Geometry: final body of the model. Coordinates: model frame, mm. Face numbers are marked on the shaded views. A direction names the side the tool comes from. Round coordinates to 2 decimals unless told otherwise and drop trailing zeros. Order: outer loops, then holes, each group sorted by start corner. A loop starts at its lowest first (then second) coordinate and runs counter-clockwise, first axis right, second up. Notation, with made-up numbers: (54.25, -18) - (110.25, -18) arc R23 ccw to (110.25, 8) - close; hole circle Ø10 at (67, -4). An arc over 180 degrees is marked (long way). Put each result on its own line as item: value. Start each with the question number.
(1) Section C-C (z = -10.5). Output: boundary loops of the cut face in (x, y), and give its area (3 significant figures).
(2) Pin query (flat end, axial travel): P1, Ø1, axis at x = 30, y = 8, coming from the +Z side; P2, Ø8, axis at x = 11, y = -10.5, coming from the -Z side; P3, Ø5, axis at x = 42, z = 14.5, coming from the -Y side. Return the tip coordinate at first contact, or that it passes through.
(3) Section D-D (y = -38). Output: boundary loops of the cut face in (x, z), and give its area (3 significant figures).
(4) Material intervals for L1, parallel to X at y = 11.5, z = -61.5; L2, parallel to Y at x = 41, z = 19.5; L3, parallel to Z at x = 43, y = -18, sorted ascending. Write a range as [from, to].
(5) Pull-direction query (Y, two-part tool) for the marked faces 5, 6, 7 and 8; classes: released by +Y, released by -Y, zero draft, split by the parting line, or undercut.
(6) Section B-B (x = 40). Count the separate pieces of the cut face and the enclosed holes in it, and give its area (3 significant figures).
(7) Section A-A (y = 6). Output: boundary loops of the cut face in (x, z).
(8) Access query for the marked faces 1, 2, 3 and 4. Directions: +Z, -Z, +X, -X, +Y, -Y. A direction counts if a zero-diameter tool reaches every point of the face in a straight line with its end or side. Return the directions, or none.
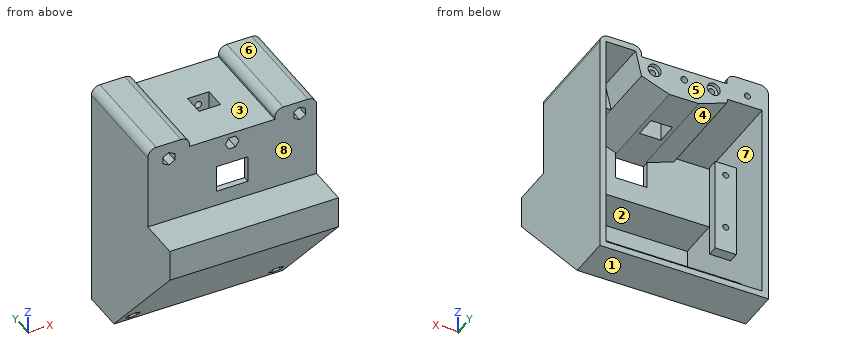
from build123d import *

# Parameters (mm, degrees)
BOSS_EXTRUDE1_DEPTH = 80
SHELL1_T            = -3
SKETCH3_W           = 46
SKETCH3_H           = 47
BOSS_EXTRUDE2_DEPTH = 17
SKETCH4_W           = 10.2
SKETCH4_H           = 10.2
CUT_EXTRUDE1_DEPTH  = 20
SKETCH6_W           = 15
SKETCH6_H           = 12.8
CUT_EXTRUDE2_DEPTH  = 3
SKETCH7_W           = 40.4
SKETCH7_H           = 50
CUT_EXTRUDE3_DEPTH  = 5
FILLET1_R           = 4
CUT_EXTRUDE7_DEPTH  = 47
SKETCH13_R          = 1.5
CUT_EXTRUDE8_DEPTH  = 25
SKETCH14_R          = 3.1
CUT_EXTRUDE9_DEPTH  = 2
SKETCH17_W          = 45
SKETCH17_H          = 5
BOSS_EXTRUDE5_DEPTH = 74
CUT_EXTRUDE10_REACH = 126.093
SKETCH18_W          = 54
SKETCH18_H          = 45
CUT_EXTRUDE11_REACH = 126.093
SKETCH19_R          = 1.45
BOSS_EXTRUDE6_DEPTH = 47
SKETCH22_R          = 1.45
CUT_EXTRUDE12_DEPTH = 135.415364765
BOSS_EXTRUDE7_DEPTH = 74
SKETCH27_R          = 1.65
CUT_EXTRUDE14_DEPTH = 10
CUT_EXTRUDE15_START = -3
CUT_EXTRUDE15_DEPTH = 32
CUT_EXTRUDE16_DEPTH = 30
BOSS_EXTRUDE8_DEPTH = 20
SKETCH31_R          = 1.5
CUT_EXTRUDE17_DEPTH = 123.649786567
CUT_EXTRUDE18_DEPTH = 15
CUT_EXTRUDE19_REACH = 126.093
SKETCH33_W          = 10
SKETCH33_H          = 5
SKETCH34_R          = 1.6
CUT_EXTRUDE20_DEPTH = 135.415364765
CUT_EXTRUDE22_DEPTH = 14


with BuildPart() as part:
    # Sketch2 → Boss-Extrude1 (new body)
    with BuildSketch(Plane(origin=(0, 0, 0), x_dir=(0, 0, -1), z_dir=(1, 0, 0))):
        Polygon((-27.320490368, 20.998248687), (-27.320490368, -29.001751313), (12.679509632, -29.001751313), (12.679509632, -48.511383538), (27.679509632, -48.511383538), (82.679509632, 0.998248687), (82.679509632, 20.998248687), align=None)
    extrude(amount=BOSS_EXTRUDE1_DEPTH)

    # Shell1
    shell1_openings = [part.faces().sort_by_distance(p)[0] for p in [
        (40, 20.998248687, -27.679509632),
    ]]
    offset(amount=SHELL1_T, openings=shell1_openings, kind=Kind.INTERSECTION)

    # Sketch3 → Boss-Extrude2 (add)
    with BuildSketch(Plane(origin=(0, 0, 24.320490368), x_dir=(-1, 0, 0), z_dir=(0, 0, -1))):
        with Locations((-40, -2.501751313)):
            Rectangle(SKETCH3_W, SKETCH3_H)
    extrude(amount=BOSS_EXTRUDE2_DEPTH)

    # Sketch4 → Cut-Extrude1 (cut)
    with BuildSketch(Plane.XY.offset(27.320490368)):
        with Locations((40, -4.001751313)):
            Rectangle(SKETCH4_W, SKETCH4_H)
    extrude(amount=-CUT_EXTRUDE1_DEPTH, mode=Mode.SUBTRACT)

    # Sketch6 → Cut-Extrude2 (cut)
    with BuildSketch(Plane.XZ.offset(29.001751313)):
        with Locations((40, 0.920490368)):
            Rectangle(SKETCH6_W, SKETCH6_H)
    extrude(amount=-CUT_EXTRUDE2_DEPTH, mode=Mode.SUBTRACT)

    # Sketch7 → Cut-Extrude3 (cut)
    with BuildSketch(Plane.XY.offset(27.320490368)):
        with Locations((40, -4.001751313)):
            Rectangle(SKETCH7_W, SKETCH7_H)
    extrude(amount=-CUT_EXTRUDE3_DEPTH, mode=Mode.SUBTRACT)

    # Fillet1
    fillet1_edges = [part.edges().sort_by_distance(p)[0] for p in [
        (80, -4.001751313, 27.320490368),
        (19.8, -4.001751313, 27.320490368),
        (0, -4.001751313, 27.320490368),
        (60.2, -4.001751313, 27.320490368),
    ]]
    fillet(fillet1_edges, radius=FILLET1_R)

    # Sketch12 → Cut-Extrude7 (cut)
    with BuildSketch(Plane(origin=(0, 20.998248687, 0), x_dir=(1, 0, 0), z_dir=(0, 1, 0))):
        Polygon((33, -7.320490368), (19.8, -12.320490368), (17, -24.320490368), (17, -7.320490368), align=None)
        Polygon((47, -7.320490368), (63, -7.320490368), (63, -24.320490368), (60.2, -12.320490368), align=None)
    extrude(amount=-CUT_EXTRUDE7_DEPTH, mode=Mode.SUBTRACT)

    # Sketch13 → Cut-Extrude8 (cut)
    with BuildSketch(Plane(origin=(0, 20.998248687, 0), x_dir=(1, 0, 0), z_dir=(0, 1, 0))):
        with Locations(Location((26, -17.320490368, 0), (0, 0, 270))):
            Circle(SKETCH13_R)
        with Locations(Location((54, -17.320490368, 0), (0, 0, 270))):
            Circle(SKETCH13_R)
    extrude(amount=-CUT_EXTRUDE8_DEPTH, mode=Mode.SUBTRACT)

    # Sketch14 → Cut-Extrude9 (cut)
    with BuildSketch(Plane(origin=(0, 20.998248687, 0), x_dir=(1, 0, 0), z_dir=(0, 1, 0))):
        with Locations(Location((26, -17.320490368, 0), (0, 0, 270))):
            Circle(SKETCH14_R)
        with Locations(Location((54, -17.320490368, 0), (0, 0, 270))):
            Circle(SKETCH14_R)
    extrude(amount=-CUT_EXTRUDE9_DEPTH, mode=Mode.SUBTRACT)

    # Sketch17 → Boss-Extrude5 (add)
    with BuildSketch(Plane.ZY.offset(-77)):
        with Locations((-23.179509632, -4.501751313)):
            Rectangle(SKETCH17_W, SKETCH17_H)
    extrude(amount=BOSS_EXTRUDE5_DEPTH)

    # Sketch18 → Cut-Extrude10 (cut, up to next)
    with BuildSketch(Plane(origin=(0, -2.001751313, 0), x_dir=(1, 0, 0), z_dir=(0, 1, 0)), mode=Mode.PRIVATE) as cut_extrude10_sk1:
        with Locations((40, 23.179509632)):
            Rectangle(SKETCH18_W, SKETCH18_H)
    cut_extrude10_tool1 = extrude(cut_extrude10_sk1.sketch, amount=-CUT_EXTRUDE10_REACH, mode=Mode.PRIVATE) & part.part
    add(cut_extrude10_tool1.solids().sort_by_distance((40, -2.001751, -23.17951))[0], mode=Mode.SUBTRACT)

    # Sketch19 → Cut-Extrude11 (cut, up to next)
    with BuildSketch(Plane(origin=(0, -2.001751313, 0), x_dir=(1, 0, 0), z_dir=(0, 1, 0)), mode=Mode.PRIVATE) as cut_extrude11_sk1:
        with Locations(Location((72, 37.179509632, 0), (0, 0, 270))):
            Circle(SKETCH19_R)
    cut_extrude11_tool1 = extrude(cut_extrude11_sk1.sketch, amount=-CUT_EXTRUDE11_REACH, mode=Mode.PRIVATE) & part.part
    # Sketch19 → Cut-Extrude11 (cut, up to next)
    with BuildSketch(Plane(origin=(0, -2.001751313, 0), x_dir=(1, 0, 0), z_dir=(0, 1, 0)), mode=Mode.PRIVATE) as cut_extrude11_sk2:
        with Locations(Location((72, 6.179509632, 0), (0, 0, 270))):
            Circle(SKETCH19_R)
    cut_extrude11_tool2 = extrude(cut_extrude11_sk2.sketch, amount=-CUT_EXTRUDE11_REACH, mode=Mode.PRIVATE) & part.part
    # Sketch19 → Cut-Extrude11 (cut, up to next)
    with BuildSketch(Plane(origin=(0, -2.001751313, 0), x_dir=(1, 0, 0), z_dir=(0, 1, 0)), mode=Mode.PRIVATE) as cut_extrude11_sk3:
        with Locations(Location((8, 33.179509632, 0), (0, 0, 270))):
            Circle(SKETCH19_R)
    cut_extrude11_tool3 = extrude(cut_extrude11_sk3.sketch, amount=-CUT_EXTRUDE11_REACH, mode=Mode.PRIVATE) & part.part
    # Sketch19 → Cut-Extrude11 (cut, up to next)
    with BuildSketch(Plane(origin=(0, -2.001751313, 0), x_dir=(1, 0, 0), z_dir=(0, 1, 0)), mode=Mode.PRIVATE) as cut_extrude11_sk4:
        with Locations(Location((8, 6.179509632, 0), (0, 0, 270))):
            Circle(SKETCH19_R)
    cut_extrude11_tool4 = extrude(cut_extrude11_sk4.sketch, amount=-CUT_EXTRUDE11_REACH, mode=Mode.PRIVATE) & part.part
    add(cut_extrude11_tool1.solids().sort_by_distance((72, -2.001751, -37.17951))[0], mode=Mode.SUBTRACT)
    add(cut_extrude11_tool2.solids().sort_by_distance((72, -2.001751, -6.17951))[0], mode=Mode.SUBTRACT)
    add(cut_extrude11_tool3.solids().sort_by_distance((8, -2.001751, -33.17951))[0], mode=Mode.SUBTRACT)
    add(cut_extrude11_tool4.solids().sort_by_distance((8, -2.001751, -6.17951))[0], mode=Mode.SUBTRACT)

    # Sketch21 → Boss-Extrude6 (add)
    with BuildSketch(Plane(origin=(0, -26.001751313, 0), x_dir=(1, 0, 0), z_dir=(0, 1, 0))):
        Polygon((3, -24.320490368), (3, -14.320490368), (19.333333333, -14.320490368), (17, -24.320490368), align=None)
    extrude(amount=BOSS_EXTRUDE6_DEPTH)

    # Sketch22 → Cut-Extrude12 (cut, through all)
    with BuildSketch(Plane(origin=(0, 20.998248687, 0), x_dir=(1, 0, 0), z_dir=(0, 1, 0))):
        with Locations(Location((10, -19.320490368, 0), (0, 0, 270))):
            Circle(SKETCH22_R)
    extrude(amount=-CUT_EXTRUDE12_DEPTH, mode=Mode.SUBTRACT)

    # Sketch26 → Boss-Extrude7 (add)
    with BuildSketch(Plane(origin=(3, 0, 0), x_dir=(0, 0, -1), z_dir=(1, 0, 0))):
        Polygon((79.679509632, 2.334161996), (63.679509632, 2.334161996), (63.679509632, -12.068640106), align=None)
    extrude(amount=BOSS_EXTRUDE7_DEPTH)

    # Sketch27 → Cut-Extrude14 (cut)
    with BuildSketch(Plane(origin=(0, 2.334161996, 0), x_dir=(1, 0, 0), z_dir=(0, 1, 0))):
        with Locations(Location((6, 76.679509632, 0), (0, 0, 270))):
            Circle(SKETCH27_R)
        with Locations(Location((74, 76.679509632, 0), (0, 0, 270))):
            Circle(SKETCH27_R)
    extrude(amount=-CUT_EXTRUDE14_DEPTH, mode=Mode.SUBTRACT)

    # Sketch28 → Cut-Extrude15 (cut)
    with BuildSketch(Plane(origin=(0, 2.334161996, 0), x_dir=(1, 0, 0), z_dir=(0, 1, 0)).offset(CUT_EXTRUDE15_START)):
        Polygon((74, 79.929509632), (71.185417438, 78.304509632), (71.185417438, 75.054509632), (74, 73.429509632), (76.814582562, 75.054509632), (76.814582562, 78.304509632), align=None)
        Polygon((6, 73.429509632), (8.814582562, 75.054509632), (8.814582562, 78.304509632), (6, 79.929509632), (3.185417438, 78.304509632), (3.185417438, 75.054509632), align=None)
    extrude(amount=-CUT_EXTRUDE15_DEPTH, mode=Mode.SUBTRACT)

    # Sketch29 → Cut-Extrude16 (cut)
    with BuildSketch(Plane.XZ.offset(29.001751313)):
        Polygon((7.185417438, 17.695490368), (10, 16.070490368), (12.814582562, 17.695490368), (12.814582562, 20.945490368), (10, 22.570490368), (7.185417438, 20.945490368), align=None)
    extrude(amount=-CUT_EXTRUDE16_DEPTH, mode=Mode.SUBTRACT)

    # Sketch30 → Boss-Extrude8 (add)
    with BuildSketch(Plane(origin=(0, -26.001751313, 0), x_dir=(1, 0, 0), z_dir=(0, 1, 0))):
        Polygon((77, -24.320490368), (63, -24.320490368), (60.2, -12.320490368), (77, -12.320490368), align=None)
    extrude(amount=BOSS_EXTRUDE8_DEPTH)

    # Sketch31 → Cut-Extrude17 (cut, through all)
    with BuildSketch(Plane(origin=(0, -6.001751313, 0), x_dir=(1, 0, 0), z_dir=(0, 1, 0))):
        with Locations(Location((72, -21.320490368, 0), (0, 0, 270))):
            Circle(SKETCH31_R)
    extrude(amount=-CUT_EXTRUDE17_DEPTH, mode=Mode.SUBTRACT)

    # Sketch32 → Cut-Extrude18 (cut)
    with BuildSketch(Plane.XZ.offset(29.001751313)):
        Polygon((72, 24.570490368), (69.185417438, 22.945490368), (69.185417438, 19.695490368), (72, 18.070490368), (74.814582562, 19.695490368), (74.814582562, 22.945490368), align=None)
    extrude(amount=-CUT_EXTRUDE18_DEPTH, mode=Mode.SUBTRACT)

    # Sketch33 → Cut-Extrude19 (cut, up to next)
    with BuildSketch(Plane(origin=(0, -2.001751313, 0), x_dir=(1, 0, 0), z_dir=(0, 1, 0)), mode=Mode.PRIVATE) as cut_extrude19_sk1:
        with Locations((72, 43.179509632)):
            Rectangle(SKETCH33_W, SKETCH33_H)
    cut_extrude19_tool1 = extrude(cut_extrude19_sk1.sketch, amount=-CUT_EXTRUDE19_REACH, mode=Mode.PRIVATE) & part.part
    add(cut_extrude19_tool1.solids().sort_by_distance((72, -2.001751, -43.17951))[0], mode=Mode.SUBTRACT)

    # Sketch34 → Cut-Extrude20 (cut, through all)
    with BuildSketch(Plane(origin=(0, 20.998248687, 0), x_dir=(1, 0, 0), z_dir=(0, 1, 0))):
        with Locations(Location((40, -17.320490368, 0), (0, 0, 270))):
            Circle(SKETCH34_R)
    extrude(amount=-CUT_EXTRUDE20_DEPTH, mode=Mode.SUBTRACT)

    # Sketch36 → Cut-Extrude22 (cut)
    with BuildSketch(Plane.XZ.offset(29.001751313)):
        Polygon((38.375, 20.13507293), (36.75, 17.320490368), (38.375, 14.505907805), (41.625, 14.505907805), (43.25, 17.320490368), (41.625, 20.13507293), align=None)
    extrude(amount=-CUT_EXTRUDE22_DEPTH, mode=Mode.SUBTRACT)


solid = part.part
Checks:
1. outline: (0, -29) - (80, -29) - (80, 21) - (77, 21) - (77, -2) - (67, -2) - (67, -7) - (77, -7) - (77, -26) - (3, -26) - (3, -7) - (13, -7) - (13, -2) - (3, -2) - (3, 21) - (0, 21) - close
1. area: 622 mm²
2. P1: stops at z = 22.32
2. P2: stops at z = -74.35
2. P3: stops at y = -29
3. outline: (0, -39.36) - (80, -39.36) - (80, -12.68) - (0, -12.68) - close; hole (3, -34.87) - (77, -34.87) - (77, -15.68) - (3, -15.68) - close
3. area: 714 mm²
4. L1: x = [0, 3], [77, 80]
4. L2: y = [-15, -9.1], [1.1, 21]
4. L3: z = [-61.57, -57.09], [7.32, 16.89], [17.75, 22.32]
5. face 5: released by +Y
5. face 6: zero draft
5. face 7: undercut
5. face 8: released by -Y
6. separate pieces: 5
6. enclosed holes: 0
6. area: 951 mm²
7. outline: (0, -82.68) - (80, -82.68) - (80, 23.32) arc R4 ccw to (76, 27.32) - (64.2, 27.32) arc R4 ccw to (60.2, 23.32) - (60.2, 22.32) - (19.8, 22.32) - (19.8, 23.32) arc R4 ccw to (15.8, 27.32) - (4, 27.32) arc R4 ccw to (0, 23.32) - close; hole (3, -79.68) - (77, -79.68) - (77, 24.32) - (63, 24.32) - (60.2, 12.32) - (47, 7.32) - (33, 7.32) - (19.8, 12.32) - (19.33, 14.32) - (3, 14.32) - close; hole circle Ø2.9 at (10, 19.32); hole circle Ø3 at (26, 17.32); hole circle Ø3.2 at (40, 17.32); hole circle Ø3 at (54, 17.32)
8. face 1: -Z, +X, -X, +Y, -Y
8. face 2: none
8. face 3: +Z, +Y, -Y
8. face 4: +Y
